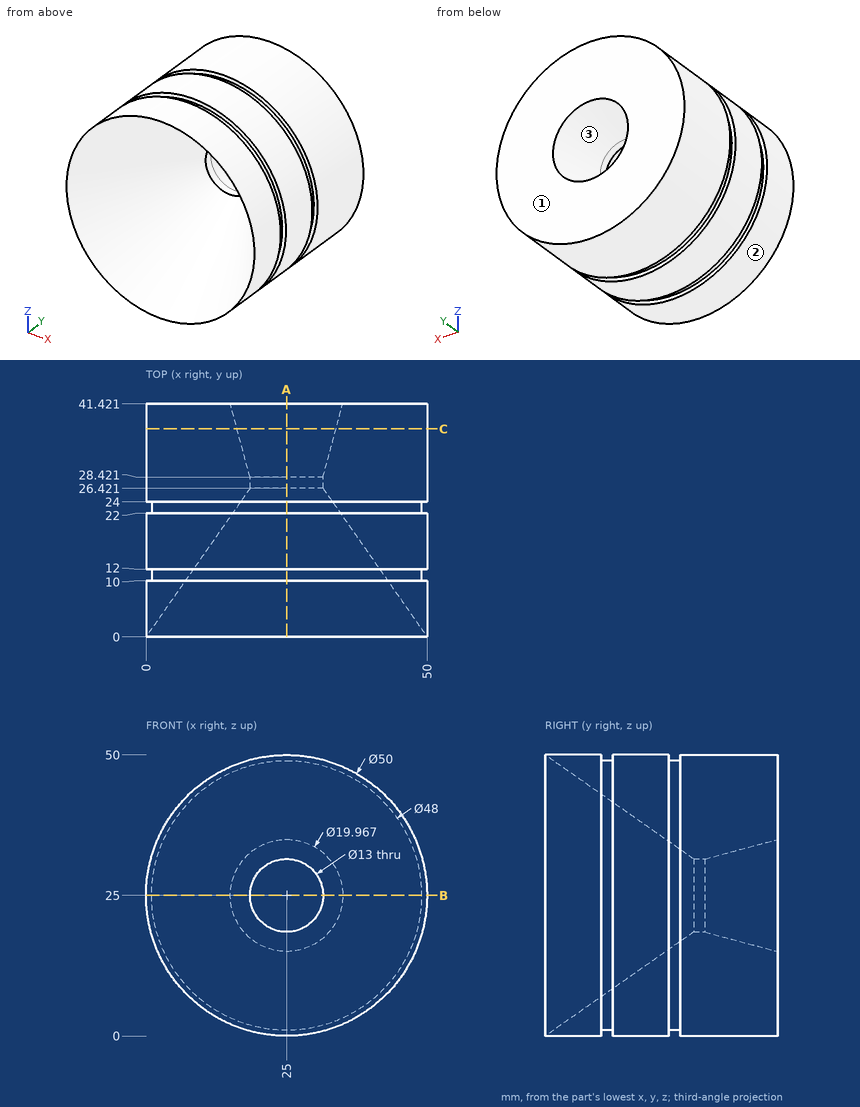
Here's the drawing with two shaded views (mm, measured from the low corner). I have some questions. Give positions to 0.01 mm unless a question says otherwise; leave off trailing zeros. Order: outer loops, then holes, each group sorted by start corner. A loop starts at its lowest first (then second) coordinate and runs counter-clockwise, first axis right, second up. Notation, with made-up numbers: M 56,81.25 L 90,81.25 A20 cw 90,117.25 Z; hole C 54.25,4 d10. An arc over 180 degrees is marked long. One line per item, written item: value.
1) I want a section at C-C, the plane y = 37. List the corners of the cut face in (x, z) for me.
Answer sheet:
outline: C 25,25 d50; hole C 25,25 d17.6
2) I want a section at A-A, the plane x = 25. List the corners of the cut face in (y, z) for me.
Answer sheet:
outline: M 0,0 L 10,0 L 10,1 L 12,1 L 12,0 L 22,0 L 22,1 L 24,1 L 24,0 L 41.42,0 L 41.42,15.02 L 28.42,18.5 L 26.42,18.5 Z; M 0,50 L 26.42,31.5 L 28.42,31.5 L 41.42,34.98 L 41.42,50 L 24,50 L 24,49 L 22,49 L 22,50 L 12,50 L 12,49 L 10,49 L 10,50 Z
3) Please list where these lines run through material, in increasing order: line 1 along X through (y, z) = (27.85, 25); line 2 along Z through (x, y) = (28.5, 3) (1 decimal); line 3 along X through (y, z) = (13, 27).
Answer sheet:
line 1: x = 0 to 18.5, 31.5 to 50
line 2: z = 0.2 to 2.4, 47.6 to 49.8
line 3: x = 0.08 to 9.23, 40.77 to 49.92
4) I want a section at B-B, the plane z = 25. List the corners of the cut face in (x, y) for me.
Answer sheet:
outline: M 0,0 L 18.5,26.42 L 18.5,28.42 L 15.02,41.42 L 0,41.42 L 0,24 L 1,24 L 1,22 L 0,22 L 0,12 L 1,12 L 1,10 L 0,10 Z; M 31.5,26.42 L 50,0 L 50,10 L 49,10 L 49,12 L 50,12 L 50,22 L 49,22 L 49,24 L 50,24 L 50,41.42 L 34.98,41.42 L 31.5,28.42 Z
5) For P1, Ø2, axis at y = 33.5, z = 14, coming from the +X side; P2, Ø10, axis at x = 32, y = 32.5, coming from the +Z side; P3, Ø6, axis at x = 18.5, y = 33.5, coming from the +Z side, each with a flat end and sliding along its axis, tell me the tip position at first contact or that it passes through.
Answer sheet:
P1: stops at x = 47.91
P2: stops at z = 49.92
P3: stops at z = 49.75
6) We'd pull the mould along Z, two halves only. Please class the marked faces 1, 2 and 3: released by +Z, released by -Z, zero draft, split by the parting line, or undercut.
Answer sheet:
face 1: zero draft
face 2: split by the parting line
face 3: undercut
